Geometry: final body of the model. Coordinates: model frame, mm. Give positions to 0.01 mm unless a question says otherwise; leave off trailing zeros. Order: outer loops, then holes, each group sorted by start corner. A loop starts at its lowest first (then second) coordinate and runs counter-clockwise, first axis right, second up. Notation, with made-up numbers: (2.5, 56.5) - (53.5, 56.5) arc R23 cw to (53.5, 75.5) - close; hole circle Ø5 at (89, -20). An arc over 180 degrees is marked (long way). One line per item, written item: value.
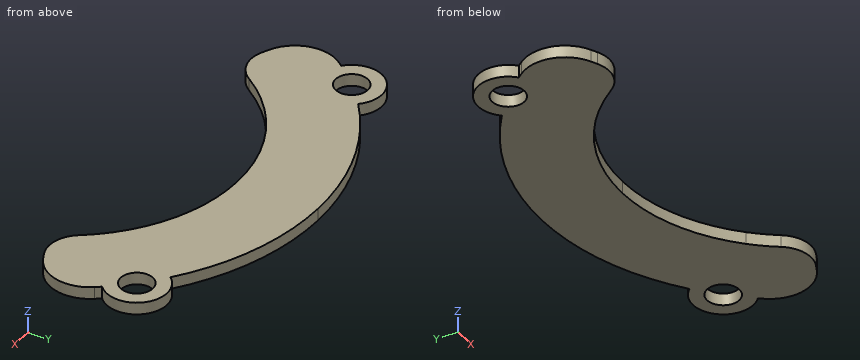
```python
from build123d import *

# Parameters (mm, degrees)
BOSS_EXTRUDE1_DEPTH = 3
SKETCH2_R           = 4
CUT_EXTRUDE1_DEPTH  = 3
SCALE1_SCALE        = 3


with BuildPart() as part:
    # Sketch1 → Boss-Extrude1 (new body)
    with BuildSketch(Plane.XY):
        with BuildLine():
            ThreePointArc((-34.913508692, 24.234209515), (-19.70147324, 37.657694462), (0, 42.5))
            Line((0, 42.5), (0, 62.5))
            ThreePointArc((0, 62.5), (-20.410075573, 59.073503494), (-38.582229462, 49.169722083))
            ThreePointArc((-38.582229462, 49.169722083), (-44.194173824, 44.194173824), (-49.169722083, 38.582229462))
            ThreePointArc((-49.169722083, 38.582229462), (-49.667032373, 37.939898462), (-50.155952108, 37.291158043))
            ThreePointArc((-50.155952108, 37.291158043), (-51.839867242, 28.929182932), (-46.459785364, 22.31005029))
            Line((-46.459785364, 22.31005029), (-44.948491744, 21.584325098))
            ThreePointArc((-44.948491744, 21.584325098), (-39.442958133, 21.061075731), (-34.913508692, 24.234209515))
        make_face()
        with BuildLine():
            ThreePointArc((0, 42.5), (16.264045876, 39.264880132), (30.0520382, 30.0520382))
            Line((30.0520382, 30.0520382), (44.194173824, 44.194173824))
            ThreePointArc((44.194173824, 44.194173824), (41.462902158, 46.766203017), (38.582229462, 49.169722083))
            ThreePointArc((38.582229462, 49.169722083), (20.410075573, 59.073503494), (0, 62.5))
            Line((0, 62.5), (0, 42.5))
        make_face()
        with BuildLine():
            Line((44.194173824, 44.194173824), (30.0520382, 30.0520382))
            ThreePointArc((30.0520382, 30.0520382), (32.612763658, 27.251745753), (34.913508692, 24.234209515))
            ThreePointArc((34.913508692, 24.234209515), (39.442958133, 21.061075731), (44.948491744, 21.584325098))
            Line((44.948491744, 21.584325098), (46.459785364, 22.31005029))
            ThreePointArc((46.459785364, 22.31005029), (51.839867242, 28.929182932), (50.155952108, 37.291158043))
            ThreePointArc((50.155952108, 37.291158043), (49.667032373, 37.939898462), (49.169722083, 38.582229462))
            ThreePointArc((49.169722083, 38.582229462), (46.766203017, 41.462902158), (44.194173824, 44.194173824))
        make_face()
        with BuildLine():
            ThreePointArc((38.582229462, 49.169722083), (41.462902158, 46.766203017), (44.194173824, 44.194173824))
            ThreePointArc((44.194173824, 44.194173824), (46.766203017, 41.462902158), (49.169722083, 38.582229462))
            ThreePointArc((49.169722083, 38.582229462), (49.497474683, 49.497474683), (38.582229462, 49.169722083))
        make_face()
        with BuildLine():
            ThreePointArc((-49.169722083, 38.582229462), (-44.194173824, 44.194173824), (-38.582229462, 49.169722083))
            ThreePointArc((-38.582229462, 49.169722083), (-49.497474683, 49.497474683), (-49.169722083, 38.582229462))
        make_face()
    extrude(amount=BOSS_EXTRUDE1_DEPTH)

    # Sketch2 → Cut-Extrude1 (cut)
    with BuildSketch(Plane.XY.offset(3)):
        with Locations((-44.194173824, 44.194173824)):
            Circle(SKETCH2_R)
        with Locations((44.194173824, 44.194173824)):
            Circle(SKETCH2_R)
    extrude(amount=-CUT_EXTRUDE1_DEPTH, mode=Mode.SUBTRACT)


with BuildPart() as part_1:
    # Scale1: scaled about (0, 43.412850072, 1.5)
    add(part.part.scale(SCALE1_SCALE).moved(Location((0, -86.825700144, -3))))


solid = part_1.part
```
1) Section A-A, the plane y = 12. Return loops of the section in (x, z).
Answers below:
outline: (-156, -3) - (-80.56, -3) - (-80.56, 6) - (-156, 6) - close; (80.56, -3) - (156, -3) - (156, 6) - (80.56, 6) - close
2) First-contact query: pin 1 (4 mm diameter, centred on y = 3.5, z = 0.5, fed in from -X); pin 2 (4 mm diameter, centred on x = -77.5, z = 0, fed in from -Y). Flat tips, straight axial feed; report the tip coordinate or a pass-through.
Answers below:
pin 1: x = -156.35
pin 2: y = 12.85
3) Material intervals for line 1 along X through (y, z) = (54, 2.5); line 2 along X through (y, z) = (-3, -1.5); line 3 along Y through (x, z) = (130, 0), sorted ascending.
Answers below:
line 1: -153.52 to -141.3, -123.86 to 123.86, 141.3 to 153.52
line 2: -154.62 to -96.07, 96.07 to 154.62
line 3: -23.79 to 34.04, 57.48 to 68.11
4) Section B-B, the plane z = 3.75. Return loops of the section in (x, y).
Answers below:
outline: (-150.47, 25.05) arc R30 ccw to (-139.38, -19.9) - (-134.85, -22.07) arc R24 ccw to (-104.74, -14.12) arc R127.5 cw to (104.74, -14.12) arc R24 ccw to (134.85, -22.07) - (139.38, -19.9) arc R30 ccw to (150.47, 25.05) arc R187.5 ccw to (147.51, 28.92) arc R22.5 ccw (long way) to (115.75, 60.68) arc R187.5 ccw to (-115.75, 60.68) arc R22.5 ccw (long way) to (-147.51, 28.92) arc R187.5 ccw to start; hole circle Ø24 at (-132.58, 45.76); hole circle Ø24 at (132.58, 45.76)
5) Section D-D, the plane x = 94. Return loops of the section in (y, z), then the cut area to 3 significant figures.
Answers below:
outline: (-0.68, -3) - (75.41, -3) - (75.41, 6) - (-0.68, 6) - close
area: 685 mm^2
6) Section C-C, the plane x = -124. Return loops of the section in (y, z).
Answers below:
outline: (-24.43, -3) - (37.37, -3) - (37.37, 6) - (-24.43, 6) - close; (54.14, -3) - (66.56, -3) - (66.56, 6) - (54.14, 6) - close
